Autodesk Inventor part; units mm, degrees
ref_plane "YZ Plane" through (0, 0, 0) normal (1, 0, 0) x (0, 1, 0)
ref_plane "XZ Plane" through (0, 0, 0) normal (0, 1, 0) x (-1, 0, 0)
ref_plane "XY Plane" through (0, 0, 0) normal (0, 0, 1) x (1, 0, 0)
sketch "Sketch1" plane through (0, 0, 0) normal (0, 1, 0) x (-1, 0, 0)
  line L0 (0, 0) -> (-5.6352, 0)
  line L1 (-5.6352, 0) -> (0, 0)
  line L2 (0, 0) -> (0, 8.7024)
  line L3 (0, -48) -> (97, -48)
  line L4 (97, -48) -> (97, 48)
  line L5 (97, 48) -> (0, 48)
  line L6 (0, 48) -> (0, -48)
  line L7 (85, -36) -> (20, -36)
  line L8 (20, -36) -> (20, 36)
  line L9 (20, 36) -> (85, 36)
  line L10 (85, 36) -> (85, -36)
  circle A0 centre (6, 33) radius 1.05
  circle A1 centre (6, -33) radius 1.05
  circle A2 centre (40, 42) radius 1.05
  circle A3 centre (91, 26) radius 1.05
  circle A4 centre (40, -42) radius 1.05
  circle A5 centre (91, -26) radius 1.05
  point P0 (0, -8.7024)
  dimension "d22" = 12
  dimension "d23" = 12
  dimension "d24" = 12
  dimension "d25" = 20
  dimension "d26" = 65
  dimension "d28" = 2.1
  dimension "d30" = 3
  dimension "d31" = 72
  dimension "d32" = 6
  dimension "d33" = 6
  dimension "d34" = 6
  dimension "d35" = 20
  dimension "d36" = 10
extrude "Extrusion1" add sketch "Sketch1" along normal blind 6
equation "\"d22\" = d23"
equation "\"d24\" = d23"
properties part number "case_back_fix" material "Acrylic, Clear"
Model file for the job. Use its own axes, mm. A direction names the side the tool comes from. Coordinates: 2 decimals unless noted, no trailing zeros. Loops run counter-clockwise (first coordinate to the right, second up) from the corner with the lowest first, then second, coordinate; pieces in that order, holes last. Notation, with made-up numbers: M 6.25,56.5 L 16.25,56.5 A25 cw 16.25,70.5 Z; hole C -1.5,72.5 d5. An arc over 180 degrees is marked long. Use CSV: the item, a comma, the result in double quotes. Start each with the question number.
1. Two-plate mould, pull along Z, no slides. Class faces 1 (the cylindrical face through (-91.97, 2.96, -25.6)), 2 (the flat face through (-49, 3, 48)), 3 (the cylindrical face through (-5.17, 2.96, -32.36)), 4 (the flat face through (0, 3, 1)): pulls with the +Z half, pulls with the -Z half, needs draft (parallel to the pull), parting line crosses it, or undercut.
2. Band-saw the part on A-A, the plane z = 21.5. List the corners of the cut face in (x, y), then the cut area to 3 significant figures.
3. Probe probe 1 along Z at (x, y) = (-91, 2.3); probe 2 along Z at (x, y) = (-6, 2); probe 3 along Z at (x, y) = (-40, 1.65). List the from-to ranges inside material, lowest first. Write a range as [from, to].
4. Tool access for faces 5 (the flat face through (-15, 0, 1)), 6 (the flat face through (-52, 3, 36)): list every direction of +Z, -Z, +X, -X, +Y, -Y with a clear straight run to the whole face (end or side of a thin tool).
5. Band-saw the part on C-C, the plane y = 4.35. List the corners of the cut face in (x, z).
6. Band-saw the part on B-B, the plane x = -71.5. List the corners of the cut face in (y, z).
Entries:
1,face 1,"undercut"
1,face 2,"pulls with the +Z half"
1,face 3,"undercut"
1,face 4,"needs draft"
2,outline,"M -97,0 L -85,0 L -85,6 L -97,6 Z; M -20,0 L 0,0 L 0,6 L -20,6 Z"
2,area,"192 mm2"
3,probe 1,"z = [-48, -27.05], [-24.95, 24.95], [27.05, 48]"
3,probe 2,"z = [-48, -34.05], [-31.95, 31.95], [34.05, 48]"
3,probe 3,"z = [-48, -43.05], [-40.95, -36], [36, 40.95], [43.05, 48]"
4,face 5,"+Z, -Z, +X, -X, -Y"
4,face 6,"+Y, -Y"
5,outline,"M -97,-48 L 0,-48 L 0,48 L -97,48 Z; hole C -91,-26 d2.1; hole C -91,26 d2.1; hole M -85,-36 L -20,-36 L -20,36 L -85,36 Z; hole C -40,-42 d2.1; hole C -40,42 d2.1; hole C -6,-33 d2.1; hole C -6,33 d2.1"
6,outline,"M 0,-48 L 6,-48 L 6,-36 L 0,-36 Z; M 0,36 L 6,36 L 6,48 L 0,48 Z"
